from build123d import *

# Parameters (mm, degrees)
BOSS_EXTRUDE1_DEPTH = 5
FILLET1_R           = 10
SHELL1_T            = -1
SKETCH4_R           = 1
CUT_EXTRUDE1_DEPTH  = 15.976807967
SKETCH5_W           = 5
SKETCH5_H           = 7
BOSS_EXTRUDE2_DEPTH = 2.5
SKETCH7_R           = 1.25
CUT_EXTRUDE3_DEPTH  = 17.98431764
FILLET4_R           = 2.5


# Some blends are built 0.0001 mm under size
with BuildPart() as part:
    # Sketch1 → Boss-Extrude1 (new body)
    with BuildSketch(Plane.XY):
        with BuildLine():
            ThreePointArc((-0.15625, 9.998779222), (-10, 0), (-0.15625, -9.998779222))
            ThreePointArc((-0.15625, -9.998779222), (-2.5, 0), (-0.15625, 9.998779222))
        make_face()
    extrude(amount=BOSS_EXTRUDE1_DEPTH)

    # Fillet1
    # the kernel refuses this fillet: 10 mm, written as the material it takes off along each edge
    with BuildSketch(Plane(origin=(0, 0, 5), x_dir=(0.9999950652018581, 0.003141587485880102, 0), z_dir=(0.003141587485880102, -0.9999950652018581, 0))) as fillet1_piece_1:
        with BuildLine():
            CenterArc((1.339745962, -10), FILLET1_R, 30, 60)
            Line((1.339745962, 0), (1.339745962, 0.2))
            Line((1.339745962, 0.2), (10, 0.2))
            Line((10, 0.2), (10.2, 0))
            ThreePointArc((10.2, 0), (10.2, -2.5), (10.173205081, -4.9))
            Line((10.173205081, -4.9), (10, -5))
        make_face()
    revolve(axis=Axis((0, 0, 5), (0, 0, 1)), revolution_arc=359.64, mode=Mode.SUBTRACT)

    # Shell1
    shell1_openings = [part.faces().sort_by_distance(p)[0] for p in [
        (-5.162614347, 0, 0),
    ]]
    offset(amount=SHELL1_T, openings=shell1_openings, kind=Kind.INTERSECTION)

    # Sketch4 → Cut-Extrude1 (cut, through all)
    with BuildSketch(Plane(origin=(0, 0, 0), x_dir=(0, 0, -1), z_dir=(1, 0, 0))):
        with Locations(Location((-2.466231233, 0, 0), (0, 0, 324.775001353))):
            Circle(SKETCH4_R)
    extrude(amount=-CUT_EXTRUDE1_DEPTH, mode=Mode.SUBTRACT)

    # Sketch5 → Boss-Extrude2 (add)
    with BuildSketch(Plane.XY):
        with Locations((-0.15625, -9.998779222)):
            Rectangle(SKETCH5_W, SKETCH5_H)
    extrude(amount=BOSS_EXTRUDE2_DEPTH)

    # Sketch7 → Cut-Extrude3 (cut, through all)
    with BuildSketch(Plane.XY.offset(2.5)):
        with Locations((-0.15625, -9.998779222)):
            Circle(SKETCH7_R)
    extrude(amount=-CUT_EXTRUDE3_DEPTH, mode=Mode.SUBTRACT)

    # Fillet4
    fillet4_edges = [part.edges().sort_by_distance(p)[0] for p in [
        (-2.65625, -13.498779222, 1.25),
        (2.34375, -13.498779222, 1.25),
        (2.34375, -6.498779222, 1.25),
    ]]
    fillet(fillet4_edges, radius=FILLET4_R - 0.0001)  # a hair under: the kernel refuses the full size


solid = part.part
Work out the finished part from the listing and answer in its coordinate system (mm). A direction names the side the tool comes from. Round coordinates to 2 decimals unless told otherwise and drop trailing zeros. Write each loop counter-clockwise with the first axis right and the second up, starting at its lowest first coordinate (ties: lowest second). Pieces come first, ordered by that corner, then holes. Notation, with made-up numbers: (9, 54) - (44, 54) arc R22 ccw to (44, 88) - close; hole circle Ø6 at (9, 14.25). An arc over 180 degrees is marked (long way). Answer in a Markdown table with one row per item. Add a question column.
1. For faces 5 (the flat face through (-2.656, -10, 2)), 6 (the flat face through (-2.656, -7, 1)), 7 (the cylindrical face through (-6.65, -0.67, 3.21)), 8 (the cylindrical face through (-1.94, -12.75, 1.27)), 9 (the flat face through (-1, -6.499, 1)), determine the directions among +Z, -Z, +X, -X, +Y, -Y from which every point of the face is accessible in a straight line to the end or side of a thin tool.
2. Find the intervals of material crossed by line 1 along X through (y, z) = (-1.75, 1.55); line 2 along Y through (x, z) = (-7.5, 0.25); line 3 along X through (y, z) = (1, 0.7), in increasing order. Write a range as from..to.
3. A cutting plane is placed at B-B, the plane y = 0. Count the separate pieces of the cut face and the enclosed holes in it, and give its area (3 significant figures).
4. The mould has two halves that part along Y. Classify faces 1 (the cylindrical face through (-0.32, -8.76, 1.27)), 2 (the cylindrical face through (1.63, -7.25, 1.27)), 3 (the flat face through (2.344, -10, 1)), 4 (the cylindrical face through (1.59, -12.79, 1.27)): +Y half, -Y half, draft (parallel to the pull), parting line (faces both ways), or undercut.
5. Given pin 1 (2 mm diameter, centred on x = -3, z = 1, fed in from +Y); pin 2 (1.5 mm diameter, centred on y = -7.5, z = 1, fed in from -X); pin 3 (1 mm diameter, centred on x = -4, y = -2.5, fed in from -Z), each flat-ended and moving along its own axis, determine where each tip first touches the part or whether it passes through.
6. A cutting plane is placed at A-A, the plane x = 0.5. Determine the outline of the cut face in (y, z).
Worked out:
| question | item | result |
|---|---|---|
| 1 | face 5 | +Z, -X, -Y |
| 1 | face 6 | -Z |
| 1 | face 7 | +X, -X |
| 1 | face 8 | +Z, -Z, -X, -Y |
| 1 | face 9 | +Z, -Z, +X |
| 2 | line 1 | -8.72..-7.31, -3.43..-2.43 |
| 2 | line 2 | -6.39..-4.31, 4.31..6.39 |
| 2 | line 3 | -9.5..-8.24, -3.48..-2.48 |
| 3 | separate pieces | 3 |
| 3 | enclosed holes | 0 |
| 3 | area | 6.96 mm^2 |
| 4 | face 1 | undercut |
| 4 | face 2 | +Y half |
| 4 | face 3 | draft |
| 4 | face 4 | -Y half |
| 5 | pin 1 | y = 9.61 |
| 5 | pin 2 | x = -6.76 |
| 5 | pin 3 | z = 3.12 |
| 6 | outline | (-13.41, 0) - (-11.06, 0) - (-11.06, 2.5) - (-13.41, 2.5) - close; (-8.93, 0) - (-6.59, 0) - (-6.59, 2.5) - (-8.93, 2.5) - close |
